Could you check a few things on this model? Use its own coordinates, in mm. A direction names the side the tool comes from. Give positions to 0.01 mm unless a question says otherwise; leave off trailing zeros. Write each loop counter-clockwise with the first axis right and the second up, starting at its lowest first coordinate (ties: lowest second). Pieces come first, ordered by that corner, then holes. Notation, with made-up numbers: (87.25, 11.25) - (98.25, 11.25) arc R30 cw to (98.25, 40.25) - close; hole circle Ø9 at (-20, 73). An arc over 180 degrees is marked (long way). Answer as CSV lines item,"result". Start each with the question number.
Q1. Will these pins go through, and if not, where does the flat tip stop? pin 1 Ø2.5 at (x, y) = (65.5, -2) entering from +Z; pin 2 Ø2.5 at (y, z) = (-3.5, 22.5) entering from +X; pin 3 Ø2.5 at (y, z) = (-2.5, -22.5) entering from -X.
Q2. If I drill on line 1 along X through (y, z) = (-2.1, -20.5); line 2 along Z through (x, y) = (25, -2.1); line 3 along Z through (x, y) = (14, -4.2), over which ranges is the centre line in solid material (lowest first)?
Q3. Imagine slicing it at A-A on z = 20.5. List the corners of the cut face in (x, y) for me.
Q4. On a 3-axis mill with a long thin cutter (end or side, diameter ignored), from which of +Z, -Z, +X, -X, +Y, -Y can I reach the whole of each face in a straight line? I mean faces 1 (the face through (69, -3, 19.05)), 2 (the face through (-14.356, -3, 22)), 3 (the face through (-69, -3, -19.05)), 4 (the face through (14.351, -3, -22)), 5 (the face through (68, -3, -19.05)). Say none if no direction works.
Q5. We'd pull the mould along X, two halves only. Please class faces 6 (the face through (27, -3, -19.05)), 7 (the face through (60.96, -3, 22)), 8 (the face through (-68, -3, 19.05)): pulls with the +X half, pulls with the -X half, needs draft (parallel to the pull), parting line crosses it, or undercut.
Q6. Imagine slicing it at C-C on x = 33.5. List the corners of the cut face in (y, z) for me.
Q7. Imagine slicing it at B-B on y = -2.7. List the corners of the cut face in (x, z) for me.
```python
from build123d import *

# Parameters (mm, degrees)
F0_W     = 21.2041994
F0_H     = 5.08
F0_W_2   = 24.7952006
F0_W_3   = 25.1206
F0_W_4   = 24.7904
F0_W_5   = 21.209
F1_DEPTH = 5.08


# Not quite as in the source:
# - a feature names something its author has since deleted; it is built from what else it names


with BuildPart() as f1:
    # F0 (on Front) → F1 (new body)
    with BuildSketch(Plane.XZ):
        Polygon((60.96, -19.05), (76.2, -19.05), (76.2, 19.05), (60.96, 19.05), (35.8394, 19.05), (10.4394, 19.05), (-14.3558006, 19.05), (-39.7558006, 19.05), (-60.96, 19.05), (-76.2, 19.05), (-76.2, -19.05), (-60.96, -19.05), (-35.8394, -19.05), (-10.4394, -19.05), (14.351, -19.05), (39.751, -19.05), align=None)
        with Locations((-50.3579003, 21.59)):
            Rectangle(F0_W, F0_H)
        with Locations((-1.9582003, 21.59)):
            Rectangle(F0_W_2, F0_H)
        with Locations((48.3997, 21.59)):
            Rectangle(F0_W_3, F0_H)
        with Locations((1.9558, -21.59)):
            Rectangle(F0_W_4, F0_H)
        with Locations((50.3555, -21.59)):
            Rectangle(F0_W_5, F0_H)
        with Locations((-48.3997, -21.59)):
            Rectangle(F0_W_3, F0_H)
    extrude(amount=F1_DEPTH)


solid = f1.part
```
Conclusion:
1,pin 1,"z = 19.05"
1,pin 2,"x = 60.96"
1,pin 3,"x = -60.96"
2,line 1,"-60.96 to -35.84, -10.44 to 14.35, 39.75 to 60.96"
2,line 2,"-19.05 to 19.05"
2,line 3,"-24.13 to 19.05"
3,outline,"(-60.96, -5.08) - (-39.76, -5.08) - (-39.76, 0) - (-60.96, 0) - close; (-14.36, -5.08) - (10.44, -5.08) - (10.44, 0) - (-14.36, 0) - close; (35.84, -5.08) - (60.96, -5.08) - (60.96, 0) - (35.84, 0) - close"
4,face 1,"+Z, +X, +Y, -Y"
4,face 2,"+Z, +Y, -Y"
4,face 3,"-Z, -X, +Y, -Y"
4,face 4,"-Z, +Y, -Y"
4,face 5,"-Z, +X, +Y, -Y"
5,face 6,"undercut"
5,face 7,"pulls with the +X half"
5,face 8,"needs draft"
6,outline,"(-5.08, -19.05) - (0, -19.05) - (0, 19.05) - (-5.08, 19.05) - close"
7,outline,"(-76.2, -19.05) - (-60.96, -19.05) - (-60.96, -24.13) - (-35.84, -24.13) - (-35.84, -19.05) - (-10.44, -19.05) - (-10.44, -24.13) - (14.35, -24.13) - (14.35, -19.05) - (39.75, -19.05) - (39.75, -24.13) - (60.96, -24.13) - (60.96, -19.05) - (76.2, -19.05) - (76.2, 19.05) - (60.96, 19.05) - (60.96, 24.13) - (35.84, 24.13) - (35.84, 19.05) - (10.44, 19.05) - (10.44, 24.13) - (-14.36, 24.13) - (-14.36, 19.05) - (-39.76, 19.05) - (-39.76, 24.13) - (-60.96, 24.13) - (-60.96, 19.05) - (-76.2, 19.05) - close"
